Autodesk Fusion 360 part; units mm, degrees
sketch "Sketch1" plane through (0, 0, 0) normal (0, 0, 1) x (1, 0, 0)
  circle A0 centre (0, 0) radius 8.2
  dimension "d1" = 16.4
extrude "Extrude1" add sketch "Sketch1" along normal blind 19
chamfer "Chamfer1" distance 0.5 angle 88.48 1 edges at (-7.6451, -2.9652, 19) measured on face at (1.6133, 1.7387, 19)
shell "Shell1" thickness 1 removed faces 1 at (1.6133, 1.7387, 0)
extrude "Extrude2" cut 1 faces at (0.4858, -2.1283, 19) along direction (0, 0, 1) blind 1
Geometry check sheet. Reference: the model listing, model coordinates, mm. A direction names the side the tool comes from. Round coordinates to 2 decimals unless told otherwise and drop trailing zeros. Write each loop counter-clockwise with the first axis right and the second up, starting at its lowest first coordinate (ties: lowest second). Pieces come first, ordered by that corner, then holes. Notation, with made-up numbers: (65.25, 28) -> (83.25, 28) arc R20 ccw to (83.25, 36) -> close; hole circle Ø2 at (-5, 45). An arc over 180 degrees is marked (long way). One line per item, written item: value. Start each with the question number.
(1) Cross-section at C-C, the plane z = 4.25. Record the cut outline in (x, y), and give its area (3 significant figures).
(2) Cross-section at A-A, the plane x = 0. Record the cut outline in (y, z).
(3) Scan lines: line 1 (Y direction, x = 0, z = 0.1); line 2 (Z direction, x = 4.5, y = 2.25); line 3 (X direction, y = -3.5, z = 8.5). Record each from-to range of solid material in increasing order. Write a range as [from, to].
(4) Cross-section at D-D, the plane z = 10.25. Record the cut outline in (x, y), and give its area (3 significant figures).
(5) Access from +Z, -Z, +X, -X, +Y, -Y to the whole of each face (thin tool, end or side, straight path). Record for faces 4 (the flat face through (0, 0, 19)), 5 (the conical face through (6.645, -2.093, 8.94)).
(6) Go/stop test with flat-tipped pins: pin 1 Ø5 at (x, z) = (-1, 8) entering from -Y; pin 2 Ø4 at (x, z) = (3, 5) entering from -Y; pin 3 Ø8 at (y, z) = (5.5, 5.5) entering from -X; pin 4 Ø8 at (x, y) = (4, -2) entering from -Z. Record where each tip stops, or that it passes through.
(7) Draft check along X on faces 1 (the flat face through (3, -7, 0)), 2 (the conical face through (-1.035, -7.886, 9.447)), 3 (the flat face through (0, 0, 18)). Enter one of: +X half, -X half, draft (parallel to the pull), parting line (faces both ways), or undercut.
(8) Cross-section at B-B, the plane y = 0. Record the cut outline in (x, z).
Answer:
1. outline: circle Ø16.18 at (0, 0); hole circle Ø14.18 at (0, 0)
1. area: 47.7 mm²
2. outline: (-8.2, 0) -> (-7.2, 0) -> (-7.2, 0.13) -> (-6.73, 18) -> (6.73, 18) -> (7.2, 0.13) -> (7.2, 0) -> (8.2, 0) -> (8.2, 0.16) -> (7.7, 19) -> (-7.7, 19) -> (-8.2, 0.16) -> close
3. line 1: [-8.2, -7.2], [7.2, 8.2]
3. line 2: [18, 19]
3. line 3: [-7.17, -6.04], [6.04, 7.17]
4. outline: circle Ø15.86 at (0, 0); hole circle Ø13.86 at (0, 0)
4. area: 46.7 mm²
5. face 4: +Z, +X, -X, +Y, -Y
5. face 5: -Z
6. pin 1: y = -8.05
6. pin 2: y = -8.01
6. pin 3: x = -7.92
6. pin 4: z = 0
7. face 1: draft
7. face 2: parting line
7. face 3: undercut
8. outline: (-8.2, 0) -> (-7.2, 0) -> (-7.2, 0.13) -> (-6.73, 18) -> (6.73, 18) -> (7.2, 0.16) -> (7.2, 0) -> (8.2, 0) -> (8.2, 0.16) -> (7.7, 19) -> (-7.7, 19) -> (-8.2, 0.16) -> close
